Input: part model. Units: mm. Frame: model coordinates. A direction names the side the tool comes from. Coordinates: 2 decimals unless noted, no trailing zeros. Order: outer loops, then holes, each group sorted by start corner. A loop starts at its lowest first (then second) coordinate and runs counter-clockwise, first axis right, second up. Notation, with made-up numbers: M 84.5,32.5 L 93.5,32.5 A17 cw 93.5,46.5 Z; hole C 62,20 d5. An arc over 180 degrees is marked long. One line per item, written item: value.
```python
from build123d import *

# Parameters (mm, degrees)
EXTRUDE1_DEPTH          = 2.794
HOLE1_D                 = 1.459992
HOLE1_CBORE_D           = 1.89992
HOLE1_CBORE_DEPTH       = 0.89408
EXTRUDE2_DEPTH          = 2.794
HOLE_PATTERN_COUNT      = 32
HOLE_PATTERN_PITCH      = 2.54
HOLE_PATTERN_COUNT_DIR2 = 2
HOLE_PATTERN_PITCH_DIR2 = 2.54
SLOT_PATTERN_COUNT      = 31
SLOT_PATTERN_PITCH      = 2.54


with BuildPart() as part:
    # Sketch1 → Extrude1 (new body)
    with BuildSketch(Plane(origin=(0, 0, 0), x_dir=(1, 0, 0), z_dir=(0, 1, 0))):
        Polygon((14.934373708, 0.40005), (14.774353708, 0.40005), (14.628747416, 0), (0, 0), (-0.145606292, 0.40005), (-0.305626292, 0.40005), (-0.305626292, 4.67995), (-0.145606292, 4.67995), (0, 5.08), (14.628747416, 5.08), (14.774353708, 4.67995), (14.934373708, 4.67995), align=None)
    extrude(amount=-EXTRUDE1_DEPTH)

    # Hole1 (through all)
    with Locations(Plane(origin=(0.964373708, 0, -1.27), x_dir=(0, 0, 1), z_dir=(0, 1, 0))):
        with Locations((0, 0)):
            hole1 = CounterBoreHole(HOLE1_D / 2, HOLE1_CBORE_D / 2, HOLE1_CBORE_DEPTH)

    # Sketch4 → Extrude2 (cut)
    with BuildSketch(Plane(origin=(0, 0, 0), x_dir=(1, 0, 0), z_dir=(0, 1, 0))):
        Polygon((1.928772816, 0), (2.5399746, 0), (2.394368308, 0.40005), (2.074379108, 0.40005), align=None)
        Polygon((2.074379108, 4.67995), (2.394368308, 4.67995), (2.5399746, 5.08), (1.928772816, 5.08), align=None)
    extrude2 = extrude(amount=-EXTRUDE2_DEPTH, mode=Mode.SUBTRACT)

    # Hole Pattern: Hole1 32 × 2
    with Locations(*[(i * HOLE_PATTERN_PITCH, 0, -j * HOLE_PATTERN_PITCH_DIR2) for i in range(HOLE_PATTERN_COUNT) for j in range(HOLE_PATTERN_COUNT_DIR2) if (i, j) != (0, 0)]):
        add(hole1, mode=Mode.SUBTRACT)

    # Slot Pattern: Extrude2 ×31
    with Locations(*[(i * SLOT_PATTERN_PITCH, 0, 0) for i in range(1, SLOT_PATTERN_COUNT)]):
        add(extrude2, mode=Mode.SUBTRACT)


solid = part.part
```
(1) Access query for faces 1 (the flat face through (-0.306, -1, -3)), 2 (the cylindrical face through (1.25, -0.441, -2.904)). Directions: +Z, -Z, +X, -X, +Y, -Y. A direction counts if a zero-diameter tool reaches every point of the face in a straight line with its end or side. Return the directions, or none.
Data:
face 1: +Z, -Z, -X, +Y, -Y
face 2: +Y
(2) First-contact query: pin 1 (0.6 mm diameter, centred on x = 1, z = -1, fed in from +Y); pin 2 (0.6 mm diameter, centred on x = 3, z = -3.5, fed in from +Y). Flat tips, straight axial feed; report the tip coordinate or a pass-through.
Data:
pin 1: passes through
pin 2: stops at y = -0.89
(3) Ray query, line 1 (Z direction, x = 3.25, y = -2.3); line 2 (X direction, y = -0.95, z = -0.35); line 3 (X direction, y = -1, z = -4.8). Return the intervals inside material, ascending. Write a range as from..to.
Data:
line 1: z = -5.08..-4.49, -3.13..-1.95, -0.59..0
line 2: x = -0.13..2.06, 2.41..4.6, 4.95..7.14, 7.49..9.68, 10.03..12.22, 12.57..14.76
line 3: x = -0.1..2.03, 2.44..4.57, 4.98..7.11, 7.52..9.65, 10.06..12.19, 12.6..14.73
(4) Cut plane A-A on x = 3. Output: boundary loops of the cut face in (y, z) (3 decimals), plus the area to 3 significant figures.
Data:
outline: M -2.794,-5.08 L 0,-5.08 L 0,-4.615 L -0.894,-4.615 L -0.894,-4.338 L -2.794,-4.338 Z; M -2.794,-3.282 L -0.894,-3.282 L -0.894,-3.005 L 0,-3.005 L 0,-2.075 L -0.894,-2.075 L -0.894,-1.798 L -2.794,-1.798 Z; M -2.794,-0.742 L -0.894,-0.742 L -0.894,-0.465 L 0,-0.465 L 0,0 L -2.794,0 Z
area: 7.30 mm2
(5) Draft query along Z for faces 3 (the flat face through (14.934, -1, -3)), 4 (the flat face through (4, -1, 0)), 5 (the flat face through (14, -1, -5.08)), 6 (the cylindrical face through (6.845, -0.441, -3.299)). Return one class per face: released by +Z, released by -Z, zero draft, split by the parting line, or undercut.
Data:
face 3: zero draft
face 4: released by +Z
face 5: released by -Z
face 6: undercut
(6) Cut plane B-B on z = -1.27. Give the number of separate pieces and of enclosed holes in the cut face, plus the area to 3 significant figures.
Data:
separate pieces: 7
enclosed holes: 0
area: 15.7 mm2
